Verification items for the finished model (mm, model axes). Face numbers are marked on the shaded views. A direction names the side the tool comes from. Coordinates: 2 decimals unless noted, no trailing zeros. Order: outer loops, then holes, each group sorted by start corner. A loop starts at its lowest first (then second) coordinate and runs counter-clockwise, first axis right, second up. Notation, with made-up numbers: M -35.5,-40 L 13.5,-40 A19 ccw 13.5,-13 Z; hole C 56.5,-23.75 d10. An arc over 180 degrees is marked long. Return JSON: item names as keys, results as strings. Group by question number.
Q1. Section check C-C, the plane x = -13. Enter the section's corners in (y, z).
Q2. Mould release check, pull along Z, two halves, no side actions. Record for the marked faces 4, 5 and 6: pulls with the +Z half, pulls with the -Z half, needs draft (parallel to the pull), parting line crosses it, or undercut.
Q3. Go/stop test with flat-tipped pins: pin 1 Ø1 at (x, y) = (5.5, 1.5) entering from +Z; pin 2 Ø4 at (x, z) = (-6, 1) entering from +Y; pin 3 Ø4 at (x, z) = (-7, 1) entering from -Y. Record where each tip stops, or that it passes through.
Q4. Access from +Z, -Z, +X, -X, +Y, -Y to the whole of each face (thin tool, end or side, straight path). Record for the marked faces 1, 2 and 3.
Q5. Section check D-D, the plane y = -2.5. Enter the section's corners in (x, z).
Q6. Thickness scan on probe 1 along Y at (x, z) = (-5.5, 0); probe 2 along Y at (x, z) = (-13, 0); probe 3 along X at (y, z) = (-2, 0.75). Record the ranges inside material, lowest first.
Q7. Section check A-A, the plane z = 0. Enter the section's corners in (x, y).
Q8. Section check B-B, the plane y = -0.75. Enter the section's corners in (x, z), then the cut area to 3 significant figures.
from build123d import *


with BuildPart() as f1:
    # F0 (on Front) → F1 (revolve)
    with BuildSketch(Plane.XZ):
        Polygon((-13.619311, 2.2), (-19.119311, 2.2), (-19.119311, 0), (8.980689, 0), (8.980689, 2.2), (-12.019311, 2.2), (-12.019311, 3.5), (-13.619311, 3.5), align=None)
    revolve(axis=Axis((-4.034162, 0, 0), (1, 0, 0)))

    # F2 (on Front) → F3 (revolve, cut)
    with BuildSketch(Plane.XZ):
        Polygon((-13.465806, 2), (-19.465806, 2), (-19.465806, 0), (10.834194, 0), (10.834194, 2), (-12.165806, 2), (-12.165806, 3.2), (-13.465806, 3.2), align=None)
    revolve(axis=Axis((-4.82097, 0, 0), (-1, 0, 0)), mode=Mode.SUBTRACT)


solid = f1.part
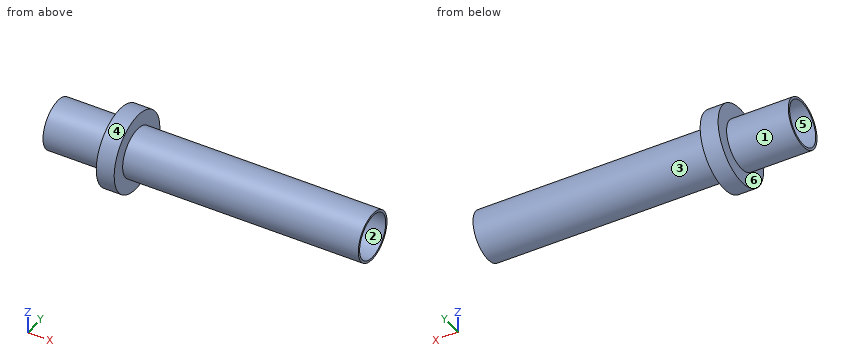
Numbers:
{
 "1": {"outline": "C 0,0 d7; hole C 0,0 d6.4"},
 "2": {"face 4": "parting line crosses it", "face 5": "undercut", "face 6": "needs draft"},
 "3": {"pin 1": "stops at z = 1.96", "pin 2": "stops at y = 2.2", "pin 3": "stops at y = -2.2"},
 "4": {"face 1": "-X", "face 2": "+X, -X", "face 3": "+X"},
 "5": {"outline": "M -13.62,-2.45 L -12.02,-2.45 L -12.02,2.45 L -13.62,2.45 Z; hole M -13.47,-2 L -12.17,-2 L -12.17,2 L -13.47,2 Z"},
 "6": {"probe 1": "y = -2.2 to -2, 2 to 2.2", "probe 2": "y = -3.5 to -3.2, 3.2 to 3.5", "probe 3": "x = -19.12 to -13.47, -12.17 to 8.98"},
 "7": {"outline": "M -19.12,-2.2 L -13.62,-2.2 L -13.62,-3.5 L -12.02,-3.5 L -12.02,-2.2 L 8.98,-2.2 L 8.98,-2 L -12.17,-2 L -12.17,-3.2 L -13.47,-3.2 L -13.47,-2 L -19.12,-2 Z; M -19.12,2 L -13.47,2 L -13.47,3.2 L -12.17,3.2 L -12.17,2 L 8.98,2 L 8.98,2.2 L -12.02,2.2 L -12.02,3.5 L -13.62,3.5 L -13.62,2.2 L -19.12,2.2 Z"},
 "8": {"outline": "M -19.12,-2.07 L -13.62,-2.07 L -13.62,-3.42 L -12.02,-3.42 L -12.02,-2.07 L 8.98,-2.07 L 8.98,-1.85 L -12.17,-1.85 L -12.17,-3.11 L -13.47,-3.11 L -13.47,-1.85 L -19.12,-1.85 Z; M -19.12,1.85 L -13.47,1.85 L -13.47,3.11 L -12.17,3.11 L -12.17,1.85 L 8.98,1.85 L 8.98,2.07 L -12.02,2.07 L -12.02,3.42 L -13.62,3.42 L -13.62,2.07 L -19.12,2.07 Z", "area": "13.1 mm2"}
}
